Geometry: see drawing. Coordinates: mm, zero at the bounding-box minimum. Give positions to 0.01 mm unless a question says otherwise; leave off trailing zeros. Order: outer loops, then holes, each group sorted by start corner. A loop starts at its lowest first (then second) coordinate and runs counter-clockwise, first axis right, second up. Notation, with made-up numbers: (-23, 38) - (8, 38) arc R17 cw to (8, 44) - close; hole circle Ø10 at (-5.75, -27.5). An arc over 180 degrees is marked (long way). Write each question's results on one line, items separated by ' | '. Start each with the question number.
Item 1: Contact query for flat-ended pins moving along their axis: pin 1 Ø4 at (x, z) = (3, 8) entering from +Y; pin 2 Ø5 at (x, z) = (8, 2.5) entering from -Y; pin 3 Ø3.5 at (y, z) = (4.74, 4.74) entering from +X. Output: stop coordinate, or through.
Item 2: Section B-B on z = 4.5. State how many separate pieces and enclosed holes the cut face has.
Item 3: Mould query, pull axis X, two halves, no side actions, for the marked faces 1, 2 and 3. Classes: released by +X, released by -X, zero draft, split by the parting line, or undercut.
Item 4: Section C-C on x = 4.5. Output: boundary loops of the cut face in (y, z) (1 decimal).
Item 5: Line query: line 1 along Z through (x, y) = (5.5, 4.75) (1 decimal); line 2 along X through (y, z) = (6.5, 0.75) (1 decimal); line 3 along Z through (x, y) = (12.5, 7.75) (1 decimal). Output: solid intervals per line, ascending.
Item 6: Section D-D on x = 10.75. Output: boundary loops of the cut face in (y, z) (1 decimal).
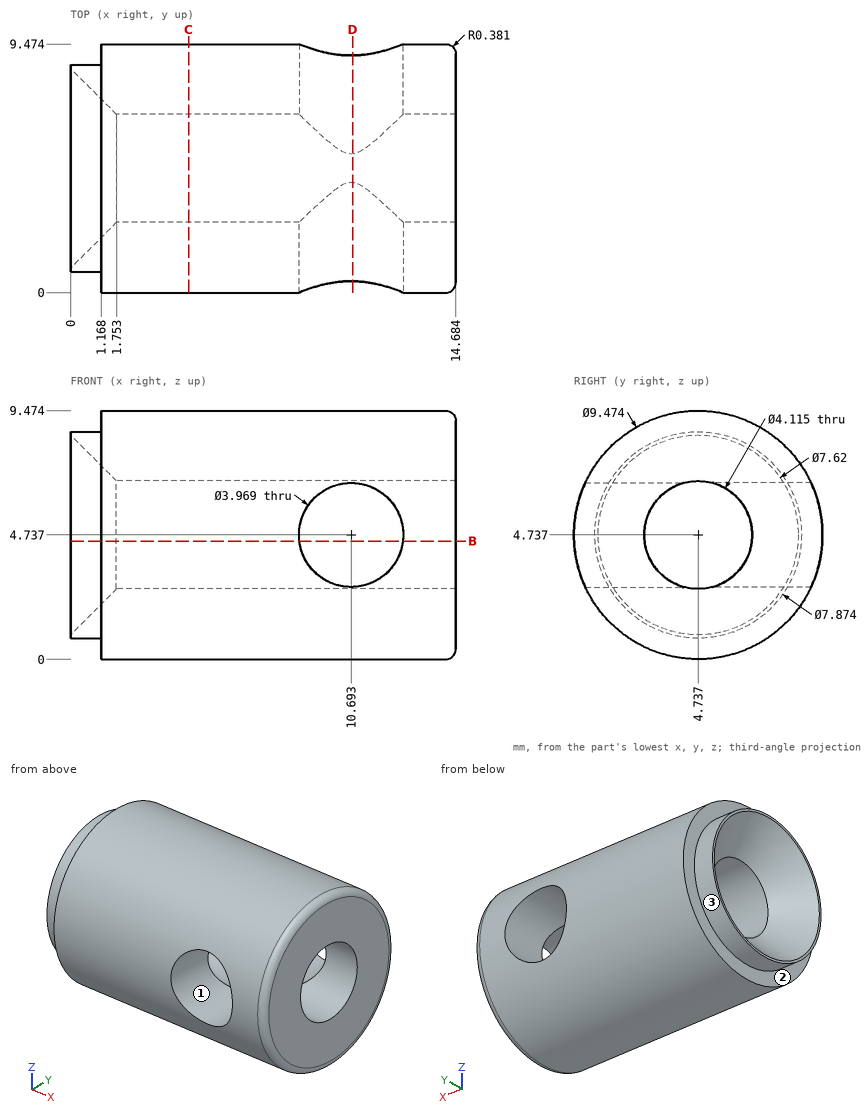
Evaluation:
1) pin 1: stops at y = 9.3 | pin 2: stops at y = 0 | pin 3: passes through
2) separate pieces: 4 | enclosed holes: 0
3) face 1: undercut | face 2: released by -X | face 3: zero draft
4) outline: circle Ø9.5 at (4.7, 4.7); hole circle Ø4.1 at (4.7, 4.7)
5) line 1: z = 0 to 2.7, 6.8 to 9.5 | line 2: x = 1.2 to 14.7 | line 3: z = 1.1 to 3.9, 5.6 to 8.4
6) outline: (0.4, 2.8) arc R4.7 ccw to (9, 2.8) - (5.3, 2.8) arc R2.1 cw to (4.2, 2.8) - close; (0.4, 6.7) - (4.2, 6.7) arc R2.1 cw to (5.3, 6.7) - (9, 6.7) arc R4.7 ccw to start
